from build123d import *

# Parameters (mm, degrees)
SZKIC1_W                    = 80
SZKIC1_H                    = 80
DODANIE_WYCI_GNI_CIE1_DEPTH = 12
SZKIC2_R                    = 15
WYTNIJ_WYCI_GNI_CIE1_DEPTH  = 6
LUSTRO2_COPY_1_SKETCH_R     = 15
LUSTRO2_COPY_1_DEPTH        = 6
ZAOKR_GLENIE1_R             = 2
SZKIC8_R                    = 2
WYTNIJ_WYCI_GNI_CIE2_DEPTH  = 58.827329179
WYTNIJ_WYCI_GNI_CIE3_DEPTH  = 3
ZAOKR_GLENIE2_R             = 0.5
SZKIC10_R                   = 32.5
DODANIE_WYCI_GNI_CIE2_DEPTH = 0.5
ZAOKR_GLENIE3_R             = 0.5
SZKIC11_R                   = 7
WYTNIJ_WYCI_GNI_CIE4_DEPTH  = 58.933151131
SFAZOWANIE1_SIZE            = 0.5
DODANIE_WYCI_GNI_CIE3_START = 128
SZKIC12_R                   = 7
SZKIC12_R_2                 = 2
DODANIE_WYCI_GNI_CIE3_DEPTH = 128
DODANIE_WYCI_GNI_CIE4_START = 12
DODANIE_WYCI_GNI_CIE4_DEPTH = 12
SZKIC16_W                   = 12
SZKIC16_H                   = 8
DODANIE_WYCI_GNI_CIE5_DEPTH = 3
SZKIC17_R                   = 2
DODANIE_WYCI_GNI_CIE6_DEPTH = 5


with BuildPart() as part:
    # Szkic1 → Dodanie-wyciągnięcie1 (new body)
    with BuildSketch(Plane(origin=(0, 0, 0), x_dir=(1, 0, 0), z_dir=(0, 1, 0))):
        Rectangle(SZKIC1_W, SZKIC1_H)
    extrude(amount=DODANIE_WYCI_GNI_CIE1_DEPTH)

    # Szkic2 → Wytnij-wyciągnięcie1 (cut)
    with BuildSketch(Plane(origin=(0, 12, 0), x_dir=(1, 0, 0), z_dir=(0, 1, 0))):
        with Locations((-40, -40)):
            Circle(SZKIC2_R)
    wytnij_wyci_gni_cie1 = extrude(amount=-WYTNIJ_WYCI_GNI_CIE1_DEPTH, mode=Mode.SUBTRACT)

    # Lustro1: Wytnij-wyciągnięcie1 across plane
    add(wytnij_wyci_gni_cie1.mirror(Plane(origin=(0, 0, 0), x_dir=(0, 0, 1), z_dir=(1, 0, 0))), mode=Mode.SUBTRACT)

    # Lustro2: Wytnij-wyciągnięcie1 across plane
    add(wytnij_wyci_gni_cie1.mirror(Plane.XY), mode=Mode.SUBTRACT)

    # Lustro2 copy 1 sketch → Lustro2 copy 1 (cut)
    with BuildSketch(Plane(origin=(0, 12, 0), x_dir=(-1, 0, 0), z_dir=(0, 1, 0))):
        with Locations((-40, -40)):
            Circle(LUSTRO2_COPY_1_SKETCH_R)
    extrude(amount=-LUSTRO2_COPY_1_DEPTH, mode=Mode.SUBTRACT)

    # Zaokrąglenie1
    zaokr_glenie1_edges = [part.edges().sort_by_distance(p)[0] for p in [
        (-40, 3, 40),
        (-40, 9, 25),
        (-25, 9, 40),
        (40, 3, 40),
        (25, 9, 40),
        (40, 9, 25),
        (40, 3, -40),
        (40, 9, -25),
        (25, 9, -40),
        (-40, 3, -40),
        (-40, 9, -25),
        (-25, 9, -40),
    ]]
    fillet(zaokr_glenie1_edges, radius=ZAOKR_GLENIE1_R)

    # Szkic5 → Pogłębienie stożkowe pod M4 Wkręt z łbem płaskim1 (revolve, cut)
    with BuildSketch(Plane(origin=(-34.403805922, 6, -34.403805922), x_dir=(0, 0, 1), z_dir=(1, 0, 0))):
        Polygon((0, 0), (0, 17.031936393), (2.25, 15.68), (2.25, 2.45), (4.7, 0), align=None)
    pog_bienie_sto_kowe_pod_m4_wkr_t_z_bem = revolve(axis=Axis((-34.403805922, 12.35, -34.403805922), (0, -1, 0)), mode=Mode.SUBTRACT)

    # Lustro3: Pogłębienie stożkowe pod M4 Wkręt z łbem płaskim1 across plane
    add(pog_bienie_sto_kowe_pod_m4_wkr_t_z_bem.mirror(Plane.XY), mode=Mode.SUBTRACT)

    # Lustro4: Pogłębienie stożkowe pod M4 Wkręt z łbem płaskim1 across plane
    add(pog_bienie_sto_kowe_pod_m4_wkr_t_z_bem.mirror(Plane(origin=(0, 0, 0), x_dir=(0, 0, 1), z_dir=(1, 0, 0))), mode=Mode.SUBTRACT)

    # Lustro4 copy 1 sketch → Lustro4 copy 1 (revolve, cut)
    with BuildSketch(Plane(origin=(34.403805922, 6, 34.403805922), x_dir=(0, 0, -1), z_dir=(-1, 0, 0))):
        Polygon((0, 0), (0, 17.031936393), (2.25, 15.68), (2.25, 2.45), (4.7, 0), align=None)
    revolve(axis=Axis((34.403805922, 12.35, 34.403805922), (0, -1, 0)), mode=Mode.SUBTRACT)

    # Szkic8 → Wytnij-wyciągnięcie2 (cut, through all)
    with BuildSketch(Plane(origin=(0, 12, 0), x_dir=(1, 0, 0), z_dir=(0, 1, 0))):
        with Locations(Location((-19.403805922, 34.403805922, 0), (0, 0, 270))):
            Circle(SZKIC8_R)
        with Locations(Location((-19.403805922, -34.403805922, 0), (0, 0, 90))):
            Circle(SZKIC8_R)
        with Locations(Location((19.403805922, 34.403805922, 0), (0, 0, 90))):
            Circle(SZKIC8_R)
        with Locations(Location((19.403805922, -34.403805922, 0), (0, 0, 270))):
            Circle(SZKIC8_R)
    extrude(amount=-WYTNIJ_WYCI_GNI_CIE2_DEPTH, mode=Mode.SUBTRACT)

    # Szkic9 → Wytnij-wyciągnięcie3 (cut)
    with BuildSketch(Plane.XZ):
        with BuildLine():
            Line((15.403805922, 34.403805922), (15.403805922, 40))
            Line((15.403805922, 40), (23.403805922, 40))
            Line((23.403805922, 40), (23.403805922, 34.403805922))
            ThreePointArc((23.403805922, 34.403805922), (19.403805922, 30.403805922), (15.403805922, 34.403805922))
        make_face()
        with BuildLine():
            Line((-23.403805922, 34.403805922), (-23.403805922, 40))
            Line((-23.403805922, 40), (-15.403805922, 40))
            Line((-15.403805922, 40), (-15.403805922, 34.403805922))
            ThreePointArc((-15.403805922, 34.403805922), (-19.403805922, 30.403805922), (-23.403805922, 34.403805922))
        make_face()
        with BuildLine():
            Line((23.403805922, -34.403805922), (23.403805922, -40))
            Line((23.403805922, -40), (15.403805922, -40))
            Line((15.403805922, -40), (15.403805922, -34.403805922))
            ThreePointArc((15.403805922, -34.403805922), (19.403805922, -30.403805922), (23.403805922, -34.403805922))
        make_face()
        with BuildLine():
            Line((-15.403805922, -34.403805922), (-15.403805922, -40))
            Line((-15.403805922, -40), (-23.403805922, -40))
            Line((-23.403805922, -40), (-23.403805922, -34.403805922))
            ThreePointArc((-23.403805922, -34.403805922), (-19.403805922, -30.403805922), (-15.403805922, -34.403805922))
        make_face()
    extrude(amount=-WYTNIJ_WYCI_GNI_CIE3_DEPTH, mode=Mode.SUBTRACT)

    # Zaokrąglenie2
    zaokr_glenie2_edges = [part.edges().sort_by_distance(p)[0] for p in [
        (-19.403805922, 0, 30.403805922),
        (-15.403805922, 0, 37.201902961),
        (-23.403805922, 0, 37.201902961),
        (-19.403805922, 3, 40),
        (-23.403805922, 1.5, 40),
        (-15.403805922, 1.5, 40),
        (19.403805922, 0, -30.403805922),
        (15.403805922, 0, -37.201902961),
        (23.403805922, 0, -37.201902961),
        (19.403805922, 3, -40),
        (23.403805922, 1.5, -40),
        (15.403805922, 1.5, -40),
        (-19.403805922, 0, -30.403805922),
        (-23.403805922, 0, -37.201902961),
        (-15.403805922, 0, -37.201902961),
        (-19.403805922, 3, -40),
        (-15.403805922, 1.5, -40),
        (-23.403805922, 1.5, -40),
        (19.403805922, 0, 30.403805922),
        (23.403805922, 0, 37.201902961),
        (15.403805922, 0, 37.201902961),
        (19.403805922, 3, 40),
        (15.403805922, 1.5, 40),
        (23.403805922, 1.5, 40),
    ]]
    fillet(zaokr_glenie2_edges, radius=ZAOKR_GLENIE2_R)

    # Szkic10 → Dodanie-wyciągnięcie2 (add)
    with BuildSketch(Plane.XZ):
        with Locations(Location((0, 0, 0), (0, 0, 90))):
            Circle(SZKIC10_R)
    extrude(amount=DODANIE_WYCI_GNI_CIE2_DEPTH)

    # Zaokrąglenie3
    zaokr_glenie3_edges = [part.edges().sort_by_distance(p)[0] for p in [
        (0, -0.5, -32.5),
    ]]
    fillet(zaokr_glenie3_edges, radius=ZAOKR_GLENIE3_R - 0.0001)  # a hair under: the kernel refuses the full size

    # Szkic11 → Wytnij-wyciągnięcie4 (cut, through all)
    with BuildSketch(Plane.XZ.offset(0.5)):
        with Locations(Location((0, 0, 0), (0, 0, 270))):
            Circle(SZKIC11_R)
    extrude(amount=-WYTNIJ_WYCI_GNI_CIE4_DEPTH, mode=Mode.SUBTRACT)

    # Sfazowanie1
    sfazowanie1_edges = [part.edges().sort_by_distance(p)[0] for p in [
        (0, -0.5, 7),
    ]]
    chamfer(sfazowanie1_edges, length=SFAZOWANIE1_SIZE)

    # Szkic12 → Dodanie-wyciągnięcie3 (add)
    with BuildSketch(Plane(origin=(0, 12, 0), x_dir=(1, 0, 0), z_dir=(0, 1, 0)).offset(DODANIE_WYCI_GNI_CIE3_START)):
        with BuildLine():
            Line((-40, 23.118056984), (-40, -23.118056984))
            ThreePointArc((-40, -23.118056984), (-39.495090003, -24.446479312), (-38.235294118, -25.104167927))
            ThreePointArc((-38.235294118, -25.104167927), (-29.393398282, -29.393398282), (-25.104167927, -38.235294118))
            ThreePointArc((-25.104167927, -38.235294118), (-24.446479312, -39.495090003), (-23.118056984, -40))
            Line((-23.118056984, -40), (23.118056984, -40))
            ThreePointArc((23.118056984, -40), (24.446479312, -39.495090003), (25.104167927, -38.235294118))
            ThreePointArc((25.104167927, -38.235294118), (29.393398282, -29.393398282), (38.235294118, -25.104167927))
            ThreePointArc((38.235294118, -25.104167927), (39.495090003, -24.446479312), (40, -23.118056984))
            Line((40, -23.118056984), (40, 23.118056984))
            ThreePointArc((40, 23.118056984), (39.495090003, 24.446479312), (38.235294118, 25.104167927))
            ThreePointArc((38.235294118, 25.104167927), (29.393398282, 29.393398282), (25.104167927, 38.235294118))
            ThreePointArc((25.104167927, 38.235294118), (24.446479312, 39.495090003), (23.118056984, 40))
            Line((23.118056984, 40), (-23.118056984, 40))
            ThreePointArc((-23.118056984, 40), (-24.446479312, 39.495090003), (-25.104167927, 38.235294118))
            ThreePointArc((-25.104167927, 38.235294118), (-29.393398282, 29.393398282), (-38.235294118, 25.104167927))
            ThreePointArc((-38.235294118, 25.104167927), (-39.495090003, 24.446479312), (-40, 23.118056984))
        make_face()
        with Locations(Location((0, 0, 0), (0, 0, 90))):
            Circle(SZKIC12_R, mode=Mode.SUBTRACT)
        with Locations(Location((-19.403805922, -34.403805922, 0), (0, 0, 270))):
            Circle(SZKIC12_R_2, mode=Mode.SUBTRACT)
        with Locations(Location((19.403805922, -34.403805922, 0), (0, 0, 270))):
            Circle(SZKIC12_R_2, mode=Mode.SUBTRACT)
        with Locations(Location((19.403805922, 34.403805922, 0), (0, 0, 270))):
            Circle(SZKIC12_R_2, mode=Mode.SUBTRACT)
        with Locations(Location((-19.403805922, 34.403805922, 0), (0, 0, 270))):
            Circle(SZKIC12_R_2, mode=Mode.SUBTRACT)
    extrude(amount=-DODANIE_WYCI_GNI_CIE3_DEPTH)

    # Szkic15 → Dodanie-wyciągnięcie4 (add)
    with BuildSketch(Plane(origin=(0, 140, 0), x_dir=(1, 0, 0), z_dir=(0, 1, 0)).offset(DODANIE_WYCI_GNI_CIE4_START)):
        with BuildLine():
            Line((-40, 23.118056984), (-40, -23.118056984))
            ThreePointArc((-40, -23.118056984), (-39.495090003, -24.446479312), (-38.235294118, -25.104167927))
            ThreePointArc((-38.235294118, -25.104167927), (-29.393398282, -29.393398282), (-25.104167927, -38.235294118))
            ThreePointArc((-25.104167927, -38.235294118), (-24.446479312, -39.495090003), (-23.118056984, -40))
            Line((-23.118056984, -40), (23.118056984, -40))
            ThreePointArc((23.118056984, -40), (24.446479312, -39.495090003), (25.104167927, -38.235294118))
            ThreePointArc((25.104167927, -38.235294118), (29.393398282, -29.393398282), (38.235294118, -25.104167927))
            ThreePointArc((38.235294118, -25.104167927), (39.495090003, -24.446479312), (40, -23.118056984))
            Line((40, -23.118056984), (40, 23.118056984))
            ThreePointArc((40, 23.118056984), (39.495090003, 24.446479312), (38.235294118, 25.104167927))
            ThreePointArc((38.235294118, 25.104167927), (29.393398282, 29.393398282), (25.104167927, 38.235294118))
            ThreePointArc((25.104167927, 38.235294118), (24.446479312, 39.495090003), (23.118056984, 40))
            Line((23.118056984, 40), (-23.118056984, 40))
            ThreePointArc((-23.118056984, 40), (-24.446479312, 39.495090003), (-25.104167927, 38.235294118))
            ThreePointArc((-25.104167927, 38.235294118), (-29.393398282, 29.393398282), (-38.235294118, 25.104167927))
            ThreePointArc((-38.235294118, 25.104167927), (-39.495090003, 24.446479312), (-40, 23.118056984))
        make_face()
    extrude(amount=-DODANIE_WYCI_GNI_CIE4_DEPTH)

    # Szkic16 → Dodanie-wyciągnięcie5 (add)
    with BuildSketch(Plane(origin=(0, 0, -40), x_dir=(-1, 0, 0), z_dir=(0, 0, -1))):
        with Locations((0, 144)):
            Rectangle(SZKIC16_W, SZKIC16_H)
    extrude(amount=DODANIE_WYCI_GNI_CIE5_DEPTH)

    # Szkic17 → Dodanie-wyciągnięcie6 (add)
    with BuildSketch(Plane(origin=(0, 0, -43), x_dir=(-1, 0, 0), z_dir=(0, 0, -1))):
        with Locations((0, 144)):
            Circle(SZKIC17_R)
    extrude(amount=DODANIE_WYCI_GNI_CIE6_DEPTH)


solid = part.part
Input: part model. Units: mm. Frame: model coordinates. A direction names the side the tool comes from. Coordinates: 2 decimals unless noted, no trailing zeros. Loops run counter-clockwise (first coordinate to the right, second up) from the corner with the lowest first, then second, coordinate; pieces in that order, holes last. Notation, with made-up numbers: (39.5, -4) - (94.5, -4) arc R21 ccw to (94.5, 29) - close; hole circle Ø11 at (61, 18.5). An arc over 180 degrees is marked (long way). Answer in a Markdown table with one row per item. Add a question column.
Item 1: Section query B-B on y = 36.5. Return the cut outline in (x, z), then the cut area to 3 significant figures.
Item 2: Access query for faces 1 (the flat face through (0, 140, 0)), 2 (the cylindrical face through (-33.035, 1.8, -36.189)), 3 (the flat face through (33.6, 6, -29.6)), 4 (the flat face through (-19, 3, 37)). Directions: +Z, -Z, +X, -X, +Y, -Y. A direction counts if a zero-diameter tool reaches every point of the face in a straight line with its end or side. Return the directions, or none.
Item 3: Mould query, pull axis X, two halves, no side actions, for faces 5 (the flat face through (19, 3, -37)), 6 (the flat face through (-33.6, 6, -29.6)), 7 (the cylindrical face through (29.493, 80.022, -29.295)). Classes: released by +X, released by -X, zero draft, split by the parting line, or undercut.
Item 4: Section query C-C on y = 144. Return the cut outline in (x, z), then the cut area to 3 significant figures.
Item 5: Line query: line 1 along X through (y, z) = (71.5, 0); line 2 along X through (y, z) = (64, -36); line 3 along X through (y, z) = (43.5, 34.5). Output: solid intervals per line, ascending. Write a range as [from, to].
Item 6: Contact query for flat-ended pins moving along their axis: P1, Ø6.5, axis at x = -18.5, z = 34.5, coming from the -Y side; P2, Ø6, axis at x = 34.4, z = -34.4, coming from the -Y side; P3, Ø6, axis at y = 50, z = -37, coming from the -X side. Output: stop coordinate, or through.
Recorded:
| question | item | result |
|---|---|---|
| 1 | outline | (-40, -23.12) arc R2 ccw to (-38.24, -25.1) arc R15 cw to (-25.1, -38.24) arc R2 ccw to (-23.12, -40) - (23.12, -40) arc R2 ccw to (25.1, -38.24) arc R15 cw to (38.24, -25.1) arc R2 ccw to (40, -23.12) - (40, 23.12) arc R2 ccw to (38.24, 25.1) arc R15 cw to (25.1, 38.24) arc R2 ccw to (23.12, 40) - (-23.12, 40) arc R2 ccw to (-25.1, 38.24) arc R15 cw to (-38.24, 25.1) arc R2 ccw to (-40, 23.12) - close; hole circle Ø4 at (-19.4, -34.4); hole circle Ø4 at (-19.4, 34.4); hole circle Ø14 at (0, 0); hole circle Ø4 at (19.4, -34.4); hole circle Ø4 at (19.4, 34.4) |
| 1 | area | 5,480 mm^2 |
| 2 | face 1 | -Y |
| 2 | face 2 | +Y, -Y |
| 2 | face 3 | -Z, +X, +Y |
| 2 | face 4 | +Z, -Y |
| 3 | face 5 | undercut |
| 3 | face 6 | zero draft |
| 3 | face 7 | released by +X |
| 4 | outline | (-40, -23.12) arc R2 ccw to (-38.24, -25.1) arc R15 cw to (-25.1, -38.24) arc R2 ccw to (-23.12, -40) - (-6, -40) - (-6, -43) - (-2, -43) - (-2, -48) - (2, -48) - (2, -43) - (6, -43) - (6, -40) - (23.12, -40) arc R2 ccw to (25.1, -38.24) arc R15 cw to (38.24, -25.1) arc R2 ccw to (40, -23.12) - (40, 23.12) arc R2 ccw to (38.24, 25.1) arc R15 cw to (25.1, 38.24) arc R2 ccw to (23.12, 40) - (-23.12, 40) arc R2 ccw to (-25.1, 38.24) arc R15 cw to (-38.24, 25.1) arc R2 ccw to (-40, 23.12) - close |
| 4 | area | 5,740 mm^2 |
| 5 | line 1 | [-40, -7], [7, 40] |
| 5 | line 2 | [-25.54, -20.61], [-18.2, 18.2], [20.61, 25.54] |
| 5 | line 3 | [-26.04, -21.4], [-17.41, 17.41], [21.4, 26.04] |
| 6 | P1 | y = 0.14 |
| 6 | P2 | y = 0 |
| 6 | P3 | x = -26.25 |
